from build123d import *

# Parameters (mm, degrees)
MODEL_R             = 0.75
MODEL_W             = 9
MODEL_H             = 2
BOSS_EXTRUDE1_DEPTH = 2


with BuildPart() as part:
    # Model → Boss-Extrude1 (new body)
    with BuildSketch(Plane.XY):
        with BuildLine():
            Line((1972.109841287, 1171.284705077), (1972.109841287, 1166.284705077))
            Line((1972.109841287, 1166.284705077), (1978.109841287, 1166.284705077))
            Line((1978.109841287, 1166.284705077), (1978.109841287, 1171.284705077))
            Line((1978.109841287, 1171.284705077), (1980.109841287, 1171.284705077))
            Line((1980.109841287, 1171.284705077), (1980.109841287, 1166.284705077))
            Line((1980.109841287, 1166.284705077), (1984.109841287, 1166.284705077))
            ThreePointArc((1984.109841287, 1166.284705077), (1984.816948068, 1166.577598295), (1985.109841287, 1167.284705077))
            Line((1985.109841287, 1167.284705077), (1985.109841287, 1184.284705077))
            ThreePointArc((1985.109841287, 1184.284705077), (1984.524054849, 1185.698918639), (1983.109841287, 1186.284705077))
            Line((1983.109841287, 1186.284705077), (1967.109841287, 1186.284705077))
            ThreePointArc((1967.109841287, 1186.284705077), (1965.695627724, 1185.698918639), (1965.109841287, 1184.284705077))
            Line((1965.109841287, 1184.284705077), (1965.109841287, 1167.284705077))
            ThreePointArc((1965.109841287, 1167.284705077), (1965.402734505, 1166.577598295), (1966.109841287, 1166.284705077))
            Line((1966.109841287, 1166.284705077), (1970.109841287, 1166.284705077))
            Line((1970.109841287, 1166.284705077), (1970.109841287, 1171.284705077))
            Line((1970.109841287, 1171.284705077), (1972.109841287, 1171.284705077))
        make_face()
        with Locations((1982.359841287, 1183.784705077)):
            Circle(MODEL_R, mode=Mode.SUBTRACT)
        with Locations((1967.859841287, 1183.784705077)):
            Circle(MODEL_R, mode=Mode.SUBTRACT)
        with Locations((1982.359841287, 1178.284705077)):
            Circle(MODEL_R, mode=Mode.SUBTRACT)
        with Locations((1967.859841287, 1178.284705077)):
            Circle(MODEL_R, mode=Mode.SUBTRACT)
        with Locations((1975.109841287, 1181.284705077)):
            Rectangle(MODEL_W, MODEL_H, mode=Mode.SUBTRACT)
        with Locations((1975.109841287, 1175.284705077)):
            Rectangle(MODEL_W, MODEL_H, mode=Mode.SUBTRACT)
    extrude(amount=BOSS_EXTRUDE1_DEPTH)


solid = part.part
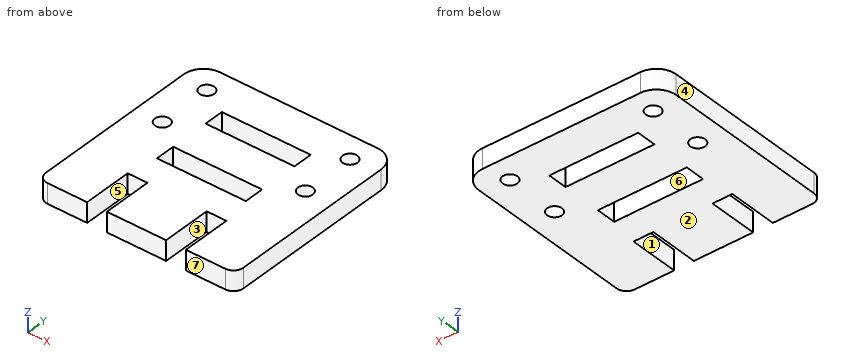
Read the model definition and answer for the solid it produces. Units are mm, in the model's axes. Face numbers are marked on the shaded views. A direction names the side the tool comes from. Round coordinates to 2 decimals unless told otherwise and drop trailing zeros. Order: outer loops, then holes, each group sorted by start corner. A loop starts at its lowest first (then second) coordinate and runs counter-clockwise, first axis right, second up.
1) The part is cut by section B-B on z = 0.3. Write down the section's boundary in (x, y), plus the area to 3 significant figures.
2) The mould has two halves that part along X. Classify the marked faces 1, 2, 3 and 4: released by +X, released by -X, zero draft, split by the parting line, or undercut.
3) The part is cut by section C-C on y = 1183.5. Write down the section's boundary in (x, z), plus the area to 3 significant figures.
4) Flat-ended cylindrical pins translate along their axes: pin 1 (2 mm diameter, centred on x = 1967.86, y = 1183.78, fed in from -Z); pin 2 (1 mm diameter, centred on x = 1971, z = 1, fed in from -Y). Find the tip coordinate at first contact, or state that the pin passes through.
5) For the marked faces 5, 6 and 7, determine the directions among +Z, -Z, +X, -X, +Y, -Y from which every point of the face is accessible in a straight line to the end or side of a thin tool.
6) The part is cut by section A-A on x = 1979. Write down the section's boundary in (y, z), plus the area to 3 significant figures.
7) Straight lines are drawn through the part: L1, parallel to X at y = 1183.75, z = 1.35; L2, parallel to Y at x = 1975, z = 1.5; L3, parallel to Y at x = 1971, z = 0.6. For each, find the intervals that lie inside material, in ascending order.
Resolved:
1. outline: (1965.11, 1167.28) arc R1 ccw to (1966.11, 1166.28) - (1970.11, 1166.28) - (1970.11, 1171.28) - (1972.11, 1171.28) - (1972.11, 1166.28) - (1978.11, 1166.28) - (1978.11, 1171.28) - (1980.11, 1171.28) - (1980.11, 1166.28) - (1984.11, 1166.28) arc R1 ccw to (1985.11, 1167.28) - (1985.11, 1184.28) arc R2 ccw to (1983.11, 1186.28) - (1967.11, 1186.28) arc R2 ccw to (1965.11, 1184.28) - close; hole circle Ø1.5 at (1967.86, 1178.28); hole circle Ø1.5 at (1967.86, 1183.78); hole (1970.61, 1174.28) - (1979.61, 1174.28) - (1979.61, 1176.28) - (1970.61, 1176.28) - close; hole (1970.61, 1180.28) - (1979.61, 1180.28) - (1979.61, 1182.28) - (1970.61, 1182.28) - close; hole circle Ø1.5 at (1982.36, 1178.28); hole circle Ø1.5 at (1982.36, 1183.78)
1. area: 335 mm2
2. face 1: undercut
2. face 2: zero draft
2. face 3: undercut
2. face 4: released by -X
3. outline: (1965.11, 0) - (1967.17, 0) - (1967.17, 2) - (1965.11, 2) - close; (1968.55, 0) - (1981.67, 0) - (1981.67, 2) - (1968.55, 2) - close; (1983.05, 0) - (1985.11, 0) - (1985.11, 2) - (1983.05, 2) - close
3. area: 34.4 mm2
4. pin 1: stops at z = 0
4. pin 2: stops at y = 1171.28
5. face 5: +Z, -Z, -Y
5. face 6: +Z, -Z
5. face 7: +Z, -Z, +X, -X, -Y
6. outline: (1171.28, 0) - (1174.28, 0) - (1174.28, 2) - (1171.28, 2) - close; (1176.28, 0) - (1180.28, 0) - (1180.28, 2) - (1176.28, 2) - close; (1182.28, 0) - (1186.28, 0) - (1186.28, 2) - (1182.28, 2) - close
6. area: 22.0 mm2
7. L1: x = 1965.11 to 1967.11, 1968.61 to 1981.61, 1983.11 to 1985.11
7. L2: y = 1166.28 to 1174.28, 1176.28 to 1180.28, 1182.28 to 1186.28
7. L3: y = 1171.28 to 1174.28, 1176.28 to 1180.28, 1182.28 to 1186.28
